```python
from build123d import *

# Parameters (mm, degrees)
ESQUISSE1_W             = 270
ESQUISSE1_H             = 160
BOSS_EXTRU_1_DEPTH      = 8
CHANFREIN1_SIZE         = 30
ESQUISSE2_W             = 40
ESQUISSE2_H             = 60
ESQUISSE2_W_2           = 10
ENL_V_MAT_EXTRU_1_DEPTH = 8
ESQUISSE3_R             = 3
BOSS_EXTRU_2_DEPTH      = 10


with BuildPart() as part:
    # Esquisse1 → Boss.-Extru.1 (new body)
    with BuildSketch(Plane.XY):
        with Locations((135, 80)):
            Rectangle(ESQUISSE1_W, ESQUISSE1_H)
    extrude(amount=BOSS_EXTRU_1_DEPTH)

    # Chanfrein1
    chanfrein1_edges = [part.edges().sort_by_distance(p)[0] for p in [
        (0, 160, 4),
        (270, 160, 4),
        (270, 0, 4),
        (0, 0, 4),
    ]]
    chamfer(chanfrein1_edges, length=CHANFREIN1_SIZE)

    # Esquisse2 → Enlèv. mat.-Extru.1 (cut)
    with BuildSketch(Plane.XY.offset(8)):
        with Locations((50, 80)):
            Rectangle(ESQUISSE2_W, ESQUISSE2_H)
        with Locations((15, 80)):
            Rectangle(ESQUISSE2_W_2, ESQUISSE2_H)
        with Locations((220, 80)):
            Rectangle(ESQUISSE2_W, ESQUISSE2_H)
        with Locations((255, 80)):
            Rectangle(ESQUISSE2_W_2, ESQUISSE2_H)
    extrude(amount=-ENL_V_MAT_EXTRU_1_DEPTH, mode=Mode.SUBTRACT)

    # Esquisse3 → Boss.-Extru.2 (add)
    with BuildSketch(Plane.XY.offset(8)):
        with Locations(Location((35, 150, 0), (0, 0, 180))):
            Circle(ESQUISSE3_R)
        with Locations(Location((85, 150, 0), (0, 0, 180))):
            Circle(ESQUISSE3_R)
        with Locations(Location((185, 150, 0), (0, 0, 180))):
            Circle(ESQUISSE3_R)
        with Locations(Location((235, 150, 0), (0, 0, 180))):
            Circle(ESQUISSE3_R)
        with Locations(Location((110, 10, 0), (0, 0, 180))):
            Circle(ESQUISSE3_R)
        with Locations(Location((160, 10, 0), (0, 0, 180))):
            Circle(ESQUISSE3_R)
    extrude(amount=BOSS_EXTRU_2_DEPTH)


solid = part.part
```
CAD build for the part. Positions are in the model's coordinates, mm. A direction names the side the tool comes from. Round coordinates to 2 decimals unless told otherwise and drop trailing zeros. Order: outer loops, then holes, each group sorted by start corner. A loop starts at its lowest first (then second) coordinate and runs counter-clockwise, first axis right, second up. Notation, with made-up numbers: (37, 28.5) -> (45, 28.5) arc R11 ccw to (45, 34.5) -> close; hole circle Ø4 at (-13, 1). An arc over 180 degrees is marked (long way). One line per question, with ' | ' between items.
Q1. Probe probe 1 along X at (y, z) = (80.5, 2.75); probe 2 along X at (y, z) = (148, 10.5); probe 3 along Z at (x, y) = (22.5, 22.5). List the from-to ranges inside material, lowest first.
Completed:
probe 1: x = 0 to 10, 20 to 30, 70 to 200, 240 to 250, 260 to 270 | probe 2: x = 32.76 to 37.24, 82.76 to 87.24, 182.76 to 187.24, 232.76 to 237.24 | probe 3: z = 0 to 8
Q2. Slice it at C-C (z = 2.75). Write the cut outline in (x, y), then the cut area to 3 significant figures.
Completed:
outline: (0, 30) -> (30, 0) -> (240, 0) -> (270, 30) -> (270, 130) -> (240, 160) -> (30, 160) -> (0, 130) -> close; hole (10, 50) -> (20, 50) -> (20, 110) -> (10, 110) -> close; hole (30, 50) -> (70, 50) -> (70, 110) -> (30, 110) -> close; hole (200, 50) -> (240, 50) -> (240, 110) -> (200, 110) -> close; hole (250, 50) -> (260, 50) -> (260, 110) -> (250, 110) -> close | area: 35,400 mm^2
Q3. Slice it at A-A (y = 100.5). Write the cut outline in (x, z).
Completed:
outline: (0, 0) -> (10, 0) -> (10, 8) -> (0, 8) -> close; (20, 0) -> (30, 0) -> (30, 8) -> (20, 8) -> close; (70, 0) -> (200, 0) -> (200, 8) -> (70, 8) -> close; (240, 0) -> (250, 0) -> (250, 8) -> (240, 8) -> close; (260, 0) -> (270, 0) -> (270, 8) -> (260, 8) -> close
Q4. Two-plate mould, pull along X, no slides. Class faces 4 (the flat face through (160, 10, 18)), 5 (the flat face through (240, 80, 4)), 6 (the flat face through (20, 80, 4)), 7 (the flat face through (255, 145, 4)): released by +X, released by -X, zero draft, split by the parting line, or undercut.
Completed:
face 4: zero draft | face 5: undercut | face 6: undercut | face 7: released by +X
Q5. Slice it at D-D (y = 10). Write the cut outline in (x, z), then the cut area to 3 significant figures.
Completed:
outline: (20, 0) -> (250, 0) -> (250, 8) -> (163, 8) -> (163, 18) -> (157, 18) -> (157, 8) -> (113, 8) -> (113, 18) -> (107, 18) -> (107, 8) -> (20, 8) -> close | area: 1,960 mm^2
Q6. Drop flat-ended pins along their axis: pin 1 (6.5 mm diameter, centred on x = 17, z = 2.5, fed in from +Y); pin 2 (6.5 mm diameter, centred on x = 257, z = 4, fed in from +Y); pin 3 (9 mm diameter, centred on x = 14, z = 5, fed in from -Y); pin 4 (10 mm diameter, centred on x = 184, z = 11.5, fed in from -Y). Give the stop position or say it passes through.
Completed:
pin 1: stops at y = 150.25 | pin 2: stops at y = 146.25 | pin 3: stops at y = 11.5 | pin 4: stops at y = 0
Q7. Which spindle directions (+Z, -Z, +X, -X, +Y, -Y) get a long thin tool onto all of the face, cutting with end or side? Do faces 1 (the cylindrical face through (87.21, 147.97, 12.93)), 2 (the flat face through (185, 150, 18)), 3 (the flat face through (70, 80, 4)). Say none if no direction does.
Completed:
face 1: +Z | face 2: +Z, +X, -X, +Y, -Y | face 3: +Z, -Z
Q8. Slice it at B-B (x = 235). Write the cut outline in (y, z), then the cut area to 3 significant figures.
Completed:
outline: (0, 0) -> (50, 0) -> (50, 8) -> (0, 8) -> close; (110, 0) -> (160, 0) -> (160, 8) -> (153, 8) -> (153, 18) -> (147, 18) -> (147, 8) -> (110, 8) -> close | area: 860 mm^2
